Autodesk Fusion 360 part; units mm, degrees
sketch "Sketch1" plane through (0, 0, 0) normal (0, 0, 1) x (1, 0, 0) in component "Shaft Cap"
  line L0 (0, 164.1124) -> (0, -164.1124) construction
  line L1 (-160, 0) -> (160, 0) construction
  line L2 (-18, -7) -> (18, -7)
  arc A0 (18, -7) -> (18, 7) centre (18, 0) ccw
  line L3 (18, 7) -> (-18, 7)
  arc A1 (-18, 7) -> (-18, -7) centre (-18, 0) ccw
  line L4 (-18, 0) -> (18, 0) construction
  circle A2 centre (-18, 0) radius 1.625
  circle A3 centre (18, 0) radius 1.625
  circle A4 centre (-18, 0) radius 4.875
  circle A5 centre (18, 0) radius 4.875
  line L5 (-14.6802, 0) -> (-16.3401, 2.875)
  line L6 (-16.3401, 2.875) -> (-19.6599, 2.875)
  line L7 (-19.6599, 2.875) -> (-21.3198, 0)
  line L8 (-21.3198, 0) -> (-19.6599, -2.875)
  line L9 (-19.6599, -2.875) -> (-16.3401, -2.875)
  line L10 (-16.3401, -2.875) -> (-14.6802, 0)
  line L11 (14.6802, 0) -> (16.3401, -2.875)
  line L12 (16.3401, -2.875) -> (19.6599, -2.875)
  line L13 (19.6599, -2.875) -> (21.3198, 0)
  line L14 (21.3198, 0) -> (19.6599, 2.875)
  line L15 (19.6599, 2.875) -> (16.3401, 2.875)
  line L16 (16.3401, 2.875) -> (14.6802, 0)
  point P0 (-18, 0)
  point P1 (18, 0)
  dimension "d1" = 14
  dimension "d2" = 36
  dimension "d3" = 3.25
  dimension "d4" = 9.75
  dimension "d5" = 5.75
extrude "Extrude1" add sketch "Sketch1" against normal blind 4 contours L2 A0 L3 A1 | A4 | A5 | L5 L6 L7 L8 L9 L10 | L11 L12 L13 L14 L15 L16 in component "Shaft Cap"
extrude "Extrude2" add sketch "Sketch1" along normal blind 2.2 contours A4 | A5 | L5 L6 L7 L8 L9 L10 | L11 L12 L13 L14 L15 L16 in component "Shaft Cap"
extrude "Extrude3" cut sketch "Sketch1" along normal blind 4 from surface at -4 contours L5 L6 L7 L8 L9 L10 | L11 L12 L13 L14 L15 L16 in component "Shaft Cap"
fillet "Fillet1" radius 0.5 4 edges at (-25, 0, 0) (0, -7, 0) (25, 0, 0) (0, 7, 0) in component "Shaft Cap"
fillet "Fillet1" radius 0.25 4 edges at (-25, 0, -4) (0, 7, -4) (25, 0, -4) (0, -7, -4) in component "Shaft Cap"
fillet "Fillet2" radius 0.25 12 edges at (-18, -2.875, -4) (-20.4898, -1.4375, -4) (-20.4898, 1.4375, -4) (-18, 2.875, -4) (-15.5102, 1.4375, -4) (-15.5102, -1.4375, -4) (18, -2.875, -4) (15.5102, -1.4375, -4) (15.5102, 1.4375, -4) (18, 2.875, -4) (20.4898, 1.4375, -4) (20.4898, -1.4375, -4) in component "Shaft Cap"
chamfer "Chamfer1" distance 0.5 angle 45 2 edges at (13.4549, -1.7629, 2.2) (-22.5451, -1.7629, 2.2) in component "Shaft Cap"
chamfer "Chamfer1" distance 0.5 angle 45 2 edges at (-19.515, 0.5876, 2.2) (16.485, 0.5876, 2.2) in component "Shaft Cap"
component "Shaft Cap" placed x (1, 0, 0) y (0, 1, 0) z (0, 0, 1) at (0, 0, 0)
Here's how the part is built. I have some questions about the finished solid (model axes, mm). A direction names the side the tool comes from. Give positions to 0.01 mm unless a question says otherwise; leave off trailing zeros. Order: outer loops, then holes, each group sorted by start corner. A loop starts at its lowest first (then second) coordinate and runs counter-clockwise, first axis right, second up. Notation, with made-up numbers: M -13,4.25 L 23,4.25 A10 cw 23,9.25 Z; hole C 89,-2 d4. An arc over 180 degrees is marked long. Use a Markdown table: item, result. Add a question column.
1. If we mould it in two halves opening along Y, with no side actions, what happens to faces 4 (the flat face through (0, -7, -2)), 5 (the cylindrical face through (-25, 0, -2)), 6 (the cylindrical face through (15.43, 1.45, -3.93))? For each: +Y half, -Y half, draft (parallel to the pull), parting line (faces both ways), or undercut.
2. Suppose I cut it at C-C (y = -0.5). Give the number of separate pieces and of enclosed holes in the cut face, and give its area (3 significant figures).
3. For pin 1 Ø1.9 at (x, y) = (18, 0) entering from +Z; pin 2 Ø4 at (x, y) = (5.5, 2.5) entering from +Z; pin 3 Ø2 at (x, z) = (-20, 0) entering from +Y; pin 4 Ø1.7 at (x, y) = (-19.5, 0.5) entering from -Z, each with a flat end and sliding along its axis, tell me the tip position at first contact or that it passes through.
4. I need wall thicknesses on probe 1 along Y at (x, z) = (-18, 0.75) (3 decimals); probe 2 along X at (y, z) = (-2.5, -2); probe 3 along Z at (x, y) = (8, -2). Which ranges of each line are inside material? Lowest first, please. Write a range as from..to.
5. Suppose I cut it at B-B (x = -7). List the corners of the cut face in (y, z) for me.
6. Suppose I cut it at A-A (z = -3). List the corners of the cut face in (x, y) for me (3 decimals), and give its area (3 significant figures).
7. On a 3-axis mill with a long thin cutter (end or side, diameter ignored), from which of +Z, -Z, +X, -X, +Y, -Y can I reach the whole of each face in a straight line? I mean faces 1 (the cylindrical face through (-16.5, 0.62, 0.84)), 2 (the cylindrical face through (-22.87, -0.21, 0.84)), 3 (the cylindrical face through (20.54, 1.5, -3.93)). Say none if no direction works.
Results list:
| question | item | result |
|---|---|---|
| 1 | face 4 | -Y half |
| 1 | face 5 | parting line |
| 1 | face 6 | undercut |
| 2 | separate pieces | 3 |
| 2 | enclosed holes | 0 |
| 2 | area | 179 mm² |
| 3 | pin 1 | passes through |
| 3 | pin 2 | stops at z = 0 |
| 3 | pin 3 | stops at y = 6.91 |
| 3 | pin 4 | stops at z = 0 |
| 4 | probe 1 | y = -4.875..-1.625, 1.625..4.875 |
| 4 | probe 2 | x = -24.54..-19.88, -16.12..16.12, 19.88..24.54 |
| 4 | probe 3 | z = -4..0 |
| 5 | outline | M -7,-3.75 A0.25 ccw -6.75,-4 L 6.75,-4 A0.25 ccw 7,-3.75 L 7,-0.5 A0.5 ccw 6.5,0 L -6.5,0 A0.5 ccw -7,-0.5 Z |
| 6 | outline | M -18,-7 L 18,-7 A7 ccw 18,7 L -18,7 A7 ccw Z; hole M -21.32,0 L -19.66,-2.875 L -16.34,-2.875 L -14.68,0 L -16.34,2.875 L -19.66,2.875 Z; hole M 14.68,0 L 16.34,-2.875 L 19.66,-2.875 L 21.32,0 L 19.66,2.875 L 16.34,2.875 Z |
| 6 | area | 601 mm² |
| 7 | face 1 | +Z, -Z |
| 7 | face 2 | +Z |
| 7 | face 3 | -Z |
